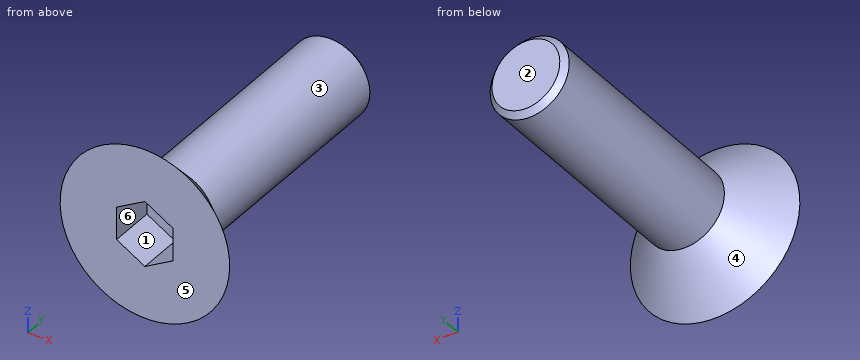
```python
from build123d import *

# Parameters (mm, degrees)
SKETCH_1_R      = 3
EXTRUDE_1_DEPTH = 1.6
CHAMFER_1_SIZE  = 1.6
SKETCH_2_R      = 1.4
EXTRUDE_2_DEPTH = 8.4
CHAMFER_2_SIZE  = 0.2


with BuildPart() as part:
    # 草图1 → 凸台-拉伸1 (new body)
    with BuildSketch(Plane(origin=(0, 0, 0), x_dir=(1, 0, 0), z_dir=(0, 1, 0))):
        with Locations(Location((0, 0, 0), (0, 0, 270))):
            Circle(SKETCH_1_R)
        Polygon((0, -1.154700538), (1, -0.577350269), (1, 0.577350269), (0, 1.154700538), (-1, 0.577350269), (-1, -0.577350269), align=None, mode=Mode.SUBTRACT)
    extrude(amount=EXTRUDE_1_DEPTH)

    # 倒角1
    # the kernel refuses this chamfer: 1.6 mm, written as the material it takes off along each edge
    with BuildSketch(Plane(origin=(0, 1.6, 0), x_dir=(0, 0, 1), z_dir=(-1, 0, 0))) as chamfer_1_piece_1:
        Polygon((3, -CHAMFER_1_SIZE), (3 - CHAMFER_1_SIZE, 0), (3, 0), align=None)
    revolve(axis=Axis((0, 1.6, 0), (0, 1, 0)), mode=Mode.SUBTRACT)

    # 草图2 → 凸台-拉伸2 (add)
    with BuildSketch(Plane(origin=(0, 1.6, 0), x_dir=(1, 0, 0), z_dir=(0, 1, 0))):
        with Locations(Location((0, 0, 0), (0, 0, 270))):
            Circle(SKETCH_2_R)
    extrude(amount=EXTRUDE_2_DEPTH)

    # 倒角2
    chamfer_2_edges = [part.edges().sort_by_distance(p)[0] for p in [
        (0, 10, -1.4),
    ]]
    chamfer(chamfer_2_edges, length=CHAMFER_2_SIZE)


solid = part.part
```
CAD build for the part. Positions are in the model's coordinates, mm. Face numbers are marked on the shaded views. A direction names the side the tool comes from. Round coordinates to 2 decimals unless told otherwise and drop trailing zeros. Write each loop counter-clockwise with the first axis right and the second up, starting at its lowest first coordinate (ties: lowest second). Pieces come first, ordered by that corner, then holes.
Item 1: Drop flat-ended pins along their axis: pin 1 Ø1 at (x, z) = (0, 0.5) entering from -Y; pin 2 Ø1.3 at (y, z) = (1, 0) entering from +X; pin 3 Ø0.6 at (y, z) = (0.5, 0) entering from -X. Give the stop position or say it passes through.
Filled in:
pin 1: stops at y = 1.6
pin 2: stops at x = 2.65
pin 3: stops at x = -2.8
Item 2: Band-saw the part on B-B on y = 8.75. Write the cut outline in (x, z).
Filled in:
outline: circle Ø2.8 at (0, 0)
Item 3: Tool access for the marked faces 1, 2 and 3: list every direction of +Z, -Z, +X, -X, +Y, -Y with a clear straight run to the whole face (end or side of a thin tool).
Filled in:
face 1: -Y
face 2: +Z, -Z, +X, -X, +Y
face 3: +Y
Item 4: Drill centre lines: L1, parallel to X at y = 7.25, z = 0; L2, parallel to Y at x = -0.1, z = 1.85; L3, parallel to Z at x = 1.15, y = 6.5. Where is each one in solid material? Low to high.
Filled in:
L1: x = -1.4 to 1.4
L2: y = 0 to 1.15
L3: z = -0.8 to 0.8
Item 5: Band-saw the part on A-A on y = 1.25. Write the cut outline in (x, z).
Filled in:
outline: circle Ø3.5 at (0, 0); hole (-1, -0.58) - (0, -1.15) - (1, -0.58) - (1, 0.58) - (0, 1.15) - (-1, 0.58) - close
Item 6: Mould opens along X. For the marked faces 4, 5 and 6 say: released by +X, released by -X, zero draft, split by the parting line, or undercut.
Filled in:
face 4: split by the parting line
face 5: zero draft
face 6: undercut
